CAD build for the part. Positions are in the model's coordinates, mm. Round coordinates to 2 decimals unless told otherwise and drop trailing zeros. Loops run counter-clockwise (first coordinate to the right, second up) from the corner with the lowest first, then second, coordinate; pieces in that order, holes last. Notation, with made-up numbers: (39.25, 46.5) - (44.25, 46.5) arc R25 cw to (44.25, 84.5) - close; hole circle Ø6 at (-6, 44.25). An arc over 180 degrees is marked (long way). One line per question, with ' | ' between items.
```python
from build123d import *

# Parameters (mm, degrees)
F4_DEPTH = 3.1
F5_DEPTH = 0.5
F6_R     = 0.25


# Not quite as in the source:
# - a feature names something its author has since deleted; it is built from what else it names


with BuildPart() as f1:
    # F0 (on Top) → F1 (revolve)
    with BuildSketch(Plane.XY):
        with BuildLine():
            Line((-14.52249, 3.1), (-13.67249, 3.1))
            Line((-13.67249, 3.1), (-13.67249, 3.95))
            ThreePointArc((-13.67249, 3.95), (-14.273530764, 3.701040764), (-14.52249, 3.1))
        make_face()
    revolve(axis=Axis((-13.67249, 1.55, 0), (0, -1, 0)))



with BuildPart() as f1b:
    # F0 (on Top) → F1, piece 2 (revolve)
    with BuildSketch(Plane.XY):
        with BuildLine():
            Line((-13.67249, -0.85), (-13.67249, 0))
            Line((-13.67249, 0), (-14.52249, 0))
            ThreePointArc((-14.52249, 0), (-14.273530764, -0.601040764), (-13.67249, -0.85))
        make_face()
    revolve(axis=Axis((-13.67249, 1.55, 0), (0, -1, 0)))


with BuildPart() as f2:
    # F0 (on Top) → F2 (revolve)
    with BuildSketch(Plane.XY):
        with BuildLine():
            Line((-0.365, 3.1), (0, 3.1))
            Line((0, 3.1), (0, 3.465))
            ThreePointArc((0, 3.465), (-0.2580939751, 3.3580939751), (-0.365, 3.1))
        make_face()
    revolve(axis=Axis((0, 1.55, 0), (0, 1, 0)))


with BuildPart() as f2b:
    # F0 (on Top) → F2, piece 2 (revolve)
    with BuildSketch(Plane.XY):
        with BuildLine():
            Line((0, -0.365), (0, 0))
            Line((0, 0), (-0.365, 0))
            ThreePointArc((-0.365, 0), (-0.2580939751, -0.2580939751), (0, -0.365))
        make_face()
    revolve(axis=Axis((0, 1.55, 0), (0, 1, 0)))


with BuildPart() as f1_1:
    add(f1.part)

    add(f1b.part)  # F4 merges F1b

    add(f2.part)  # F4 merges F2

    add(f2b.part)  # F4 merges F2b
    # F3 (on face) → F4 (join, through all)
    with BuildSketch(Plane(origin=(0, 0, 0), x_dir=(-1, 0, 0), z_dir=(0, 1, 0))):
        with BuildLine():
            Line((-1.82751, 0), (12.82249, 0))
            ThreePointArc((12.82249, 0), (13.0505296028, 0.579366261), (13.612290622, 0.847865576))
            Line((13.612290622, 0.847865576), (-1.82751, 0.3004333129))
            Line((-1.82751, 0.3004333129), (-1.82751, 0))
        make_face()
        with BuildLine():
            Line((-1.82751, -0.3004333129), (13.612290622, -0.847865576))
            ThreePointArc((13.612290622, -0.847865576), (13.0505296028, -0.579366261), (12.82249, 0))
            Line((12.82249, 0), (-1.82751, 0))
            Line((-1.82751, 0), (-1.82751, -0.3004333129))
        make_face()
        with BuildLine():
            Line((12.82249, 0), (14.52249, 0))
            ThreePointArc((14.52249, 0), (14.273530764, 0.601040764), (13.67249, 0.85))
            Line((13.67249, 0.85), (13.612290622, 0.847865576))
            ThreePointArc((13.612290622, 0.847865576), (13.0505296028, 0.579366261), (12.82249, 0))
        make_face()
        with BuildLine():
            Line((13.612290622, -0.847865576), (13.67249, -0.85))
            ThreePointArc((13.67249, -0.85), (14.273530764, -0.601040764), (14.52249, 0))
            Line((14.52249, 0), (12.82249, 0))
            ThreePointArc((12.82249, 0), (13.0505296028, -0.579366261), (13.612290622, -0.847865576))
        make_face()
    extrude(amount=F4_DEPTH)

    # F0 (on Top) → F5 (cut, symmetric)
    with BuildSketch(Plane.XY):
        with BuildLine():
            ThreePointArc((1.82751, 2.8), (0.57751, 1.55), (1.82751, 0.3))
            Line((1.82751, 0.3), (1.82751, 2.8))
        make_face()
    extrude(amount=F5_DEPTH, both=True, mode=Mode.SUBTRACT)

    # F6
    f6_edges = [f1_1.edges().sort_by_distance(p)[0] for p in [
        (0.57751, 1.55, -0.344753),
    ]]
    fillet(f6_edges, radius=F6_R)


solid = f1_1.part
```
(1) Two-plate mould, pull along X, no slides. Class faces 1 (the face through (-8, 3.1, 0)), 2 (the face through (0.578, 1.577, 0.124)): released by +X, released by -X, zero draft, split by the parting line, or undercut.
Results found:
face 1: undercut | face 2: released by +X
(2) Cut at C-C, the plane y = 3.65. Write the cut outline in (x, z).
Results found:
outline: circle Ø1.3 at (-13.67, 0)
(3) Cut at A-A, the plane z = -0.55. Write the cut outline in (x, y), then the cut area to 3 significant figures.
Results found:
outline: (-14.32, 0) arc R0.65 ccw to (-13.02, 0) - (-5.21, 0) - (-5.21, 3.1) - (-13.02, 3.1) arc R0.65 ccw to (-14.32, 3.1) - close | area: 29.6 mm²
(4) Drop flat-ended pins along their axis: P1, Ø1, axis at x = -11.5, z = 0.5, coming from the -Y side; P2, Ø2, axis at x = 0, y = 1, coming from the -Z side. Give the stop position or say it passes through.
Results found:
P1: stops at y = 0 | P2: stops at z = -0.4
(5) Cut at B-B, the plane x = -9. Write the cut outline in (y, z).
Results found:
outline: (0, -0.68) - (3.1, -0.68) - (3.1, 0.68) - (0, 0.68) - close
(6) Probe L1, parallel to Y at x = -10, z = 0.45; L2, parallel to Y at x = 1.25, z = -0.05; L3, parallel to Z at x = -9, y = 2.95. List the from-to ranges inside material, lowest first.
Results found:
L1: y = 0 to 3.1 | L2: y = 0 to 0.44, 2.66 to 3.1 | L3: z = -0.68 to 0.68
(7) Cut at D-D, the plane x = -1.5. Write the cut outline in (y, z).
Results found:
outline: (0, -0.42) - (3.1, -0.42) - (3.1, 0.42) - (0, 0.42) - close
